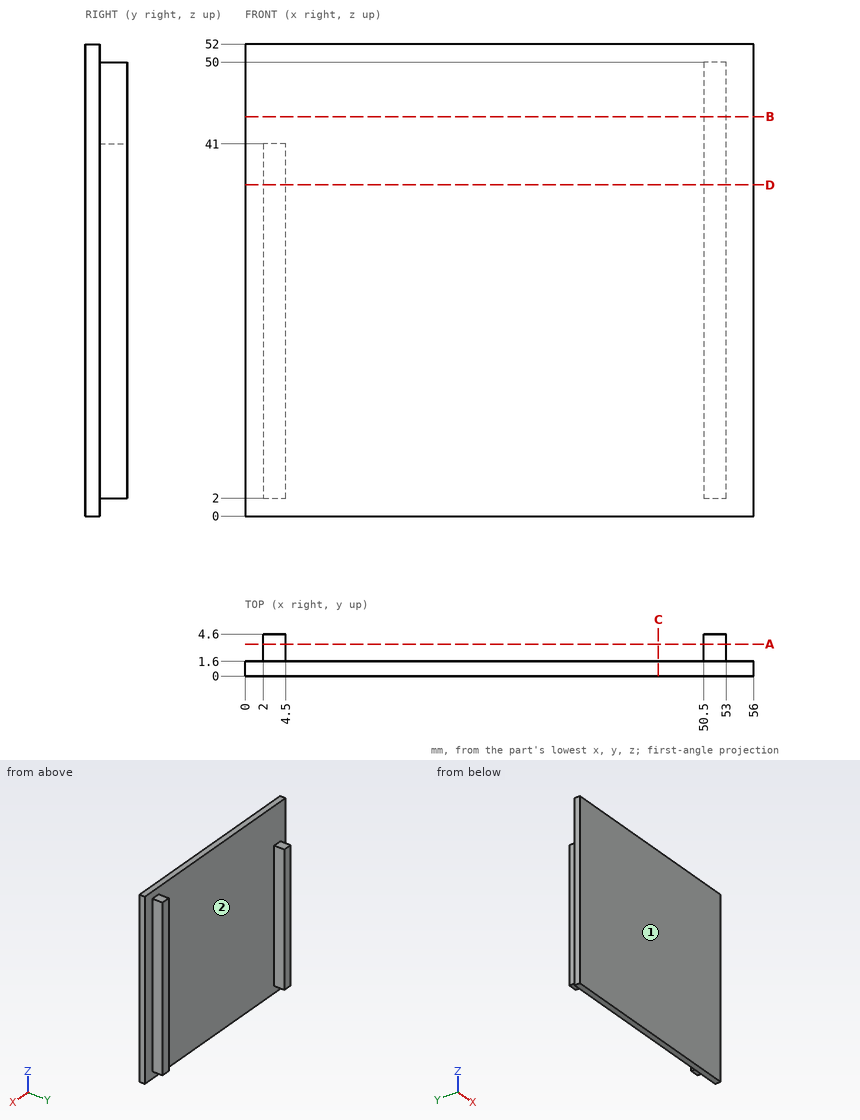
Answer from the drawing. Dimensions are ordinates in mm from the lowest x, y and z of the part. Coordinates: 2 decimals unless noted, no trailing zeros. Loops run counter-clockwise (first coordinate to the right, second up) from the corner with the lowest first, then second, coordinate; pieces in that order, holes last. Notation, with made-up numbers: (68.5, 75.25) -> (95.5, 75.25) arc R19 cw to (95.5, 86.25) -> close; hole circle Ø2 at (-40, 73.25). An arc over 180 degrees is marked (long way). Return JSON: item names as keys, results as strings.
Item 1: Find section D-D (z = 36.5). Determine the outline of the cut face in (x, y).
Answers:
{"outline": "(0, 0) -> (56, 0) -> (56, 1.6) -> (53, 1.6) -> (53, 4.6) -> (50.5, 4.6) -> (50.5, 1.6) -> (4.5, 1.6) -> (4.5, 4.6) -> (2, 4.6) -> (2, 1.6) -> (0, 1.6) -> close"}
Item 2: Find the intervals of material crossed by probe 1 along X at (y, z) = (3.2, 9); probe 2 along Y at (x, z) = (25, 40); probe 3 along X at (y, z) = (1.95, 43), in increasing order.
Answers:
{"probe 1": "x = 2 to 4.5, 50.5 to 53", "probe 2": "y = 0 to 1.6", "probe 3": "x = 50.5 to 53"}
Item 3: Flat-ended cylindrical pins translate along their axes: P1, Ø2.5, axis at y = 3.5, z = 16, coming from the +X side; P2, Ø1, axis at x = 8.5, z = 13.5, coming from the +Y side; P3, Ø2, axis at x = 51.5, y = 3.5, coming from the +Z side. Find the tip coordinate at first contact, or state that the pin passes through.
Answers:
{"P1": "stops at x = 53", "P2": "stops at y = 1.6", "P3": "stops at z = 50"}
Item 4: Find section A-A (y = 3.5). Determine the outline of the cut face in (x, z).
Answers:
{"outline": "(2, 2) -> (4.5, 2) -> (4.5, 41) -> (2, 41) -> close; (50.5, 2) -> (53, 2) -> (53, 50) -> (50.5, 50) -> close"}
Item 5: For a pull along X with two mould halves and no side action, classify the marked faces 1 and 2 as +X half, -X half, draft (parallel to the pull), parting line (faces both ways), or undercut.
Answers:
{"face 1": "draft", "face 2": "undercut"}
Item 6: Find section C-C (x = 45.5). Determine the outline of the cut face in (y, z).
Answers:
{"outline": "(0, 0) -> (1.6, 0) -> (1.6, 52) -> (0, 52) -> close"}
Item 7: Find section B-B (z = 44). Determine the outline of the cut face in (x, y), plus the area to 3 significant figures.
Answers:
{"outline": "(0, 0) -> (56, 0) -> (56, 1.6) -> (53, 1.6) -> (53, 4.6) -> (50.5, 4.6) -> (50.5, 1.6) -> (0, 1.6) -> close", "area": "97.1 mm2"}
